Autodesk Inventor part; units mm, degrees
ref_plane "YZ Plane" through (0, 0, 0) normal (1, 0, 0) x (0, 1, 0)
ref_plane "XZ Plane" through (0, 0, 0) normal (0, 1, 0) x (-1, 0, 0)
ref_plane "XY Plane" through (0, 0, 0) normal (0, 0, 1) x (1, 0, 0)
sketch "Эскиз1" plane through (0, 0, 0) normal (0, 1, 0) x (-1, 0, 0)
  line L0 (35, -85) -> (-445, -85)
  line L1 (-445, -85) -> (-445, 85)
  line L2 (-445, 85) -> (35, 85)
  line L3 (35, 85) -> (35, -85)
  point P0 (0, 0)
  point P1 (35, 0)
  dimension "d0" = 480
  dimension "d1" = 170
  dimension "d2" = 35
extrude "Выдавливание1" add sketch "Эскиз1" along normal mid plane 30
fillet "Сопряжение1" radius 30 5 edges at (445, 0, 85) (-35, 0, 85) (445, 0, -85) (-35, 0, -85) (205, 15, 85)
properties part number "Подставка1"
Geometry: final body of the model. Coordinates: model frame, mm. Coordinates: 2 decimals unless noted, no trailing zeros. Write each loop counter-clockwise with the first axis right and the second up, starting at its lowest first coordinate (ties: lowest second). Pieces come first, ordered by that corner, then holes. Notation, with made-up numbers: (14.5, 62.25) - (52.5, 62.25) arc R18 cw to (52.5, 85.25) - close; hole circle Ø1 at (-20, 86). An arc over 180 degrees is marked (long way). Return JSON: item names as keys, results as strings.
Item 1: Section query B-B (y = 2.5). Output: boundary loops of the cut face in (x, z), and give its area (3 significant figures).
Completed:
{"outline": "(-35, -55) arc R30 ccw to (-5, -85) - (415, -85) arc R30 ccw to (445, -55) - (445, 55) arc R30 ccw to (432.5, 79.37) - (-22.5, 79.37) arc R30 ccw to (-35, 55) - close", "area": "78,300 mm2"}
Item 2: Section query C-C (z = 72). Output: boundary loops of the cut face in (x, y).
Completed:
{"outline": "(-29.72, -15) - (439.72, -15) - (439.72, 9.72) - (-29.72, 9.72) - close"}
Item 3: Line query: L1, parallel to Y at x = 166.5, z = 55.5; L2, parallel to Z at x = 399.5, y = -13; L3, parallel to X at y = -3, z = 59. Output: solid intervals per line, ascending.
Completed:
{"L1": "y = -15 to 15", "L2": "z = -85 to 84.93", "L3": "x = -34.73 to 444.73"}
Item 4: Pin query (flat end, axial travel): pin 1 Ø5 at (x, y) = (168, -2.5) entering from +Z. Return the tip coordinate at first contact, or that it passes through.
Completed:
{"pin 1": "stops at z = 83.28"}
